Geometry check sheet. Reference: the model listing, model coordinates, mm. Give positions to 0.01 mm unless a question says otherwise; leave off trailing zeros. Write each loop counter-clockwise with the first axis right and the second up, starting at its lowest first coordinate (ties: lowest second). Pieces come first, ordered by that corner, then holes. Notation, with made-up numbers: (12, 59) - (57, 59) arc R28 ccw to (57, 83) - close; hole circle Ø5 at (17, 4.5). An arc over 180 degrees is marked (long way). Write item = value, one per line. Start each with the question number.
(1) Section check D-D, the plane x = 420.5. Enter the section's corners in (y, z).
(2) Section check A-A, the plane y = -90. Enter the section's corners in (x, z), plus the area to 3 significant figures.
(3) Section check C-C, the plane z = -2.25. Give the number of separate pieces and of enclosed holes in the cut face, plus the area to 3 significant figures.
(4) Depth check by flat-ended pin: pin 1 Ø1.2 at (y, z) = (-52, -12) entering from -X. Enter the tip coordinate at first touch or a pass-through.
(5) Thickness scan on L1, parallel to Y at x = 15, z = -7.25; L2, parallel to X at y = -12, z = -4.25; L3, parallel to X at y = -92.5, z = -0.75. Record the ranges inside material, lowest first.
(6) Section check B-B, the plane x = 15. Enter the section's corners in (y, z), plus the area to 3 significant figures.
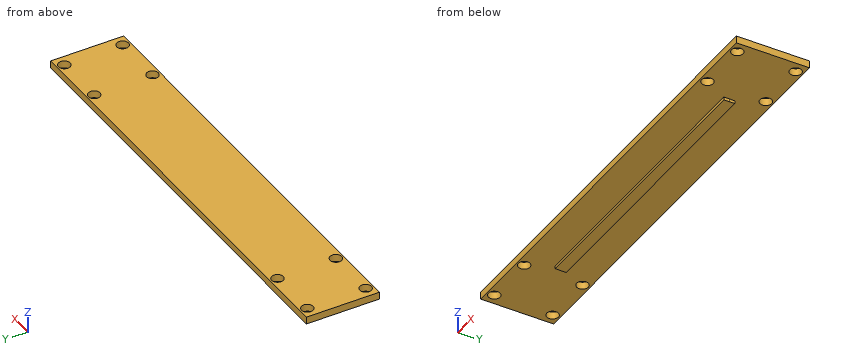
```python
from build123d import *

# Parameters (mm, degrees)
F1_DEPTH = 100
F3_D     = 16
F5_DEPTH = 4


with BuildPart() as f1:
    # F0 (on Front) → F1 (new body)
    with BuildSketch(Plane.XZ):
        Polygon((600, 0), (0, 0), (0, -10), (70, -10), (530, -10), (600, -10), align=None)
    extrude(amount=F1_DEPTH)

    # F3 (through all)
    with Locations(Plane.XY):
        with Locations((15, -10), (15, -90), (85, -10), (85, -90), (515, -10), (515, -90), (585, -90), (585, -10)):
            Hole(F3_D / 2)

    # F4 (on face) → F5 (join)
    with BuildSketch(Plane(origin=(0, 0, -10), x_dir=(1, 0, 0), z_dir=(0, 0, -1))):
        Polygon((102.29281, 57.5), (102.29281, 50), (102.29281, 42.5), (497.85471, 42.5), (497.85471, 50), (497.826087, 57.499945), align=None)
    extrude(amount=F5_DEPTH)


solid = f1.part
```
Model answer:
q1.outline = (-100, -10) - (-57.5, -10) - (-57.5, -14) - (-42.5, -14) - (-42.5, -10) - (0, -10) - (0, 0) - (-100, 0) - close
q2.outline = (0, -10) - (7, -10) - (7, 0) - (0, 0) - close; (23, -10) - (77, -10) - (77, 0) - (23, 0) - close; (93, -10) - (507, -10) - (507, 0) - (93, 0) - close; (523, -10) - (577, -10) - (577, 0) - (523, 0) - close; (593, -10) - (600, -10) - (600, 0) - (593, 0) - close
q2.area = 5,360 mm²
q3.separate_pieces = 1
q3.enclosed_holes = 8
q3.area = 58,400 mm²
q4.pin_1 = 102.29
q5.L1 = -100 to -98, -82 to -18, -2 to 0
q5.L2 = 0 to 7.25, 22.75 to 77.25, 92.75 to 507.25, 522.75 to 577.25, 592.75 to 600
q5.L3 = 0 to 7.4, 22.6 to 77.4, 92.6 to 507.4, 522.6 to 577.4, 592.6 to 600
q6.outline = (-100, -10) - (-98, -10) - (-98, 0) - (-100, 0) - close; (-82, -10) - (-18, -10) - (-18, 0) - (-82, 0) - close; (-2, -10) - (0, -10) - (0, 0) - (-2, 0) - close
q6.area = 680 mm²
